Autodesk Inventor part; units mm, degrees
ref_plane "作業平面1" through (0, 0, 4.5) normal (0, 0, 1) x (1, 0, 0)
ref_plane "YZ Plane" through (0, 0, 0) normal (1, 0, 0) x (0, 1, 0)
ref_plane "XZ Plane" through (0, 0, 0) normal (0, 1, 0) x (-1, 0, 0)
sketch "スケッチ1" plane through (0, 0, 0) normal (0, 0, 1) x (1, 0, 0)
  circle A0 centre (0, 0) radius 1.6
  circle A1 centre (0, 0) radius 3
  dimension "d0" = 3.2
  dimension "d1" = 6
extrude "押し出し1" add sketch "スケッチ1" along normal blind 2.5
sketch "スケッチ2" plane through (0, 0, 0) normal (1, 0, 0) x (0, 1, 0)
  arc A0 (2.85, 3.5) -> (-2.85, 3.5) centre (0, -0.0613) ccw
  line L0 (2.85, 3.5) -> (-2.85, 3.5)
  line L1 (-2.85, 3.5) -> (-2.85, 2.5)
  line L2 (-2.85, 2.5) -> (2.85, 2.5)
  line L3 (2.85, 2.5) -> (2.85, 3.5)
  line L4 (3, 2.5) -> (-3, 2.5)
  line L5 (10, 4.5) -> (-10, 4.5)
  line L6 (0, 2.5) -> (0, 4.5)
  point P0 (0, 0)
  point P1 (0, 4.5)
  dimension "d4" = 1
  dimension "d5" = 1
  dimension "d7" = 5.7
revolve "回転1" add sketch "スケッチ2" angle 360 about axis through (0, 0, 2.5) along (0, 0, 1) picked at (1.6112, 3.682) contours L0 L6 A0 | L3 L2 L6 L0
ref_plane "作業平面1" through (0, 0, 4.5) normal (0, 0, 1) x (1, 0, 0)
sketch "スケッチ3" plane through (0, 0, 4.5) normal (0, 0, 1) x (1, 0, 0)
  line L0 (2.25, -0.5) -> (-2.25, -0.5)
  line L1 (-2.25, -0.5) -> (-2.25, 0.5)
  line L2 (-2.25, 0.5) -> (2.25, 0.5)
  line L3 (2.25, 0.5) -> (2.25, -0.5)
  line L4 (2.25, -0.5) -> (-2.25, 0.5) construction
  line L5 (-2.25, -0.5) -> (2.25, 0.5) construction
  line L6 (-0.5, -2.25) -> (0.5, -2.25)
  line L7 (0.5, -2.25) -> (0.5, 2.25)
  line L8 (0.5, 2.25) -> (-0.5, 2.25)
  line L9 (-0.5, 2.25) -> (-0.5, -2.25)
  line L10 (-0.5, -2.25) -> (0.5, 2.25) construction
  line L11 (0.5, -2.25) -> (-0.5, 2.25) construction
  point P0 (0, 0)
  point P1 (-0.5, 0.5)
  point P2 (-0.5, -0.5)
  point P3 (0.5, -0.5)
  point P4 (0.5, 0.5)
  dimension "d9" = 4.5
  dimension "d10" = 1
extrude "押し出し2" cut sketch "スケッチ3" against normal blind 1
sketch "スケッチ5" plane through (0, 0, 2.5) normal (0, 0, 1) x (1, 0, 0)
  circle A0 centre (0, 0) radius 3
extrude "押し出し4" cut sketch "スケッチ5" along normal through all
properties part number "bearing_3_6_2.5_noscrew" material "アルミニウム 6061"
Here's how the part is built. I have some questions about the finished solid (model axes, mm). Round coordinates to 2 decimals unless told otherwise and drop trailing zeros. Order: outer loops, then holes, each group sorted by start corner. A loop starts at its lowest first (then second) coordinate and runs counter-clockwise, first axis right, second up. Notation, with made-up numbers: (-10.75, 75) -> (25.25, 75) arc R22 cw to (25.25, 113) -> close; hole circle Ø6 at (57.25, -38). An arc over 180 degrees is marked (long way). Return JSON: item names as keys, results as strings.
Q1. If we mould it in two halves opening along Y, with no side actions, what happens to faces 1 (the cylindrical face through (-1.27, 0.97, 1.23)), 2 (the flat face through (1.3, -1.3, 0)), 3 (the cylindrical face through (-3, 0, 1))? For each: released by +Y, released by -Y, zero draft, split by the parting line, or undercut.
Filled sheet:
{"face 1": "undercut", "face 2": "zero draft", "face 3": "split by the parting line"}
Q2. For pin 1 Ø1 at (x, z) = (2, 1.5) entering from -Y, with a flat end and sliding along its axis, tell me the tip position at first contact or that it passes through.
Filled sheet:
{"pin 1": "stops at y = -2.6"}
Q3. If we section it at D-D on y = 2.4: List the corners of the cut face in (x, z) for me, plus the area to 3 significant figures.
Filled sheet:
{"outline": "(-1.8, 0) -> (1.8, 0) -> (1.8, 2.5) -> (-1.8, 2.5) -> close", "area": "9.00 mm^2"}
Q4. If we section it at A-A on y = 0: List the corners of the cut face in (x, z) for me.
Filled sheet:
{"outline": "(-3, 0) -> (-1.6, 0) -> (-1.6, 2.5) -> (-3, 2.5) -> close; (1.6, 0) -> (3, 0) -> (3, 2.5) -> (1.6, 2.5) -> close"}
Q5. If we section it at C-C on z = 1.5: List the corners of the cut face in (x, y) for me, plus the area to 3 significant figures.
Filled sheet:
{"outline": "circle Ø6 at (0, 0); hole circle Ø3.2 at (0, 0)", "area": "20.2 mm^2"}
Q6. I need wall thicknesses on line 1 along Y through (x, z) = (0, 0.95); line 2 along Y through (x, z) = (-1, 0.55); line 3 along X through (y, z) = (1.3, 2.1). Which ranges of each line are inside material? Lowest first, please. Write a range as from..to.
Filled sheet:
{"line 1": "y = -3..-1.6, 1.6..3", "line 2": "y = -2.83..-1.25, 1.25..2.83", "line 3": "x = -2.7..-0.93, 0.93..2.7"}
